```python
from build123d import *

# Parameters (mm, degrees)
SKETCH2_W           = 317.094917084
SKETCH2_H           = 168.536075584
SKETCH2_R           = 4.5
SKETCH2_R_2         = 27.4955
SKETCH2_R_3         = 52.3875
SKETCH2_R_4         = 3.3
BOSS_EXTRUDE1_DEPTH = 5.715


with BuildPart() as part:
    # Sketch2 → Boss-Extrude1 (new body)
    with BuildSketch(Plane(origin=(0, 0, 0), x_dir=(1, 0, 0), z_dir=(0, 1, 0))):
        with Locations((-609.090136829, -95.384753685)):
            Rectangle(SKETCH2_W, SKETCH2_H)
        with Locations(Location((-484.179723308, -90.351987789, 0), (0, 0, 270))):
            Circle(SKETCH2_R, mode=Mode.SUBTRACT)
        with Locations(Location((-510.857294488, -90.351987789, 0), (0, 0, 270))):
            Circle(SKETCH2_R, mode=Mode.SUBTRACT)
        with Locations(Location((-463.74351815, -107.5, 0), (0, 0, 270))):
            Circle(SKETCH2_R, mode=Mode.SUBTRACT)
        with Locations(Location((-531.293499646, -107.5, 0), (0, 0, 270))):
            Circle(SKETCH2_R, mode=Mode.SUBTRACT)
        with Locations(Location((-497.518508898, -127, 0), (0, 0, 270))):
            Circle(SKETCH2_R_2, mode=Mode.SUBTRACT)
        with Locations(Location((-459.111006531, -133.772278929, 0), (0, 0, 270))):
            Circle(SKETCH2_R, mode=Mode.SUBTRACT)
        with Locations(Location((-535.926011265, -133.772278929, 0), (0, 0, 270))):
            Circle(SKETCH2_R, mode=Mode.SUBTRACT)
        with Locations(Location((-472.44979212, -156.875733282, 0), (0, 0, 270))):
            Circle(SKETCH2_R, mode=Mode.SUBTRACT)
        with Locations(Location((-522.587225676, -156.875733282, 0), (0, 0, 270))):
            Circle(SKETCH2_R, mode=Mode.SUBTRACT)
        with Locations(Location((-497.518508898, -166, 0), (0, 0, 270))):
            Circle(SKETCH2_R, mode=Mode.SUBTRACT)
        with Locations(Location((-669.29, -96.951477372, 0), (0, 0, 270))):
            Circle(SKETCH2_R_3, mode=Mode.SUBTRACT)
        with Locations(Location((-759.817588698, -19.346338398, 0), (0, 0, 270))):
            Circle(SKETCH2_R_4, mode=Mode.SUBTRACT)
        with BuildLine():
            ThreePointArc((-559.922688418, -24.132284746), (-557.312350108, -28.000893528), (-553.443741326, -25.390555218))
            ThreePointArc((-553.443741326, -25.390555218), (-556.054079636, -21.521946436), (-559.922688418, -24.132284746))
        make_face(mode=Mode.SUBTRACT)
    extrude(amount=BOSS_EXTRUDE1_DEPTH)


solid = part.part
```
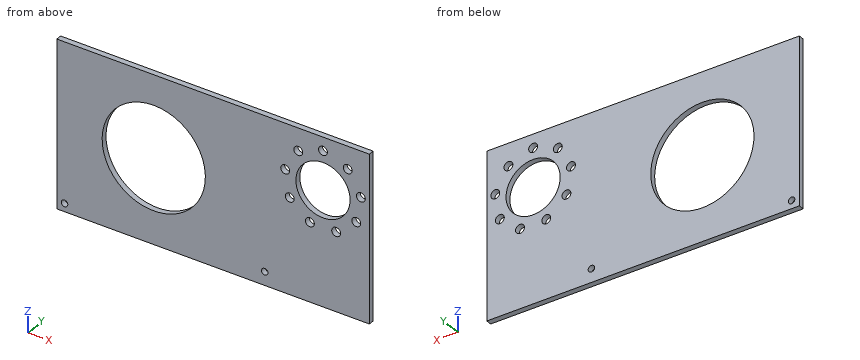
Source: CAD feature listing. Evaluate the final solid. Frame: model axes, mm. Give positions to 0.01 mm unless a question says otherwise; leave off trailing zeros. Loops run counter-clockwise (first coordinate to the right, second up) from the corner with the lowest first, then second, coordinate; pieces in that order, holes last. Notation, with made-up numbers: (-2.5, 67) -> (46.5, 67) arc R30 cw to (46.5, 93) -> close; hole circle Ø4 at (-38, 68.5). An arc over 180 degrees is marked (long way). Use a Markdown table: item, result. Add a question column.
(1) Section query C-C (y = 4.7). Count the separate pieces of the cut face and the enclosed holes in it, then the cut area to 3 significant figures.
(2) Section query D-D (z = 107.5). Output: boundary loops of the cut face in (x, y) (1 decimal).
(3) Section query B-B (x = -669.29). Output: boundary loops of the cut face in (y, z) (3 decimals), then the cut area to 3 significant figures.
(4) Section query A-A (z = 166). Output: boundary loops of the cut face in (x, y) (1 decimal), then the cut area to 3 significant figures.
(5) Ray query, line 1 (X direction, y = 1.85, z = 166); line 2 (X direction, y = 1.85, z = 19); line 3 (X direction, y = 1.2, z = 127). Return the intervals inside material, ascending.
Checked values:
| question | item | result |
|---|---|---|
| 1 | separate pieces | 1 |
| 1 | enclosed holes | 13 |
| 1 | area | 41,800 mm^2 |
| 2 | outline | (-767.6, 0) -> (-720.6, 0) -> (-720.6, 5.7) -> (-767.6, 5.7) -> close; (-618, 0) -> (-535.8, 0) -> (-535.8, 5.7) -> (-618, 5.7) -> close; (-526.8, 0) -> (-516.9, 0) -> (-516.9, 5.7) -> (-526.8, 5.7) -> close; (-478.1, 0) -> (-468.2, 0) -> (-468.2, 5.7) -> (-478.1, 5.7) -> close; (-459.2, 0) -> (-450.5, 0) -> (-450.5, 5.7) -> (-459.2, 5.7) -> close |
| 3 | outline | (0, 11.117) -> (5.715, 11.117) -> (5.715, 44.564) -> (0, 44.564) -> close; (0, 149.339) -> (5.715, 149.339) -> (5.715, 179.653) -> (0, 179.653) -> close |
| 3 | area | 364 mm^2 |
| 4 | outline | (-767.6, 0) -> (-502, 0) -> (-502, 5.7) -> (-767.6, 5.7) -> close; (-493, 0) -> (-450.5, 0) -> (-450.5, 5.7) -> (-493, 5.7) -> close |
| 4 | area | 1,760 mm^2 |
| 5 | line 1 | -767.64 to -502.02, -493.02 to -450.54 |
| 5 | line 2 | -767.64 to -763.1, -756.54 to -450.54 |
| 5 | line 3 | -767.64 to -712.2, -626.38 to -525.01, -470.02 to -450.54 |
